The listing builds one solid part. Answer for the finished solid, in the listing's coordinates (mm). Give positions to 0.01 mm unless a question says otherwise; leave off trailing zeros. Write each loop counter-clockwise with the first axis right and the second up, starting at its lowest first coordinate (ties: lowest second). Pieces come first, ordered by that corner, then holes. Notation, with made-up numbers: (34.25, -37) - (46.25, -37) arc R19 ccw to (46.25, -24) - close; hole circle Ø1 at (43.25, -19). An arc over 180 degrees is marked (long way). Write each question's results on one line, items separated by ' | '. Start each with the question number.
Q1. For a pull along X with two mould halves and no side action, classify faces 1 (the face through (0, 0, 0)), 2 (the face through (-25.81, 0.49, 16.03)) as pulls with the +X half, pulls with the -X half, needs draft (parallel to the pull), parting line crosses it, or undercut.
Q2. Find the intervals of material crossed by probe 1 along Z at (x, y) = (-27, 0.6) (3 decimals); probe 2 along Z at (x, y) = (23, 1.3); probe 3 along X at (y, z) = (1.55, 9), in increasing order.
Q3. Section A-A (x = 27) is taken. Determine the outline of the cut face in (y, z) (3 decimals).
Q4. Section C-C (z = -1) is taken. Determine the outline of the cut face in (x, y) (3 decimals).
Q5. Section B-B (y = 1.5) is taken. Determine the outline of the cut face in (x, z).
Q6. Flat-ended cylindrical pins translate along their axes: pin 1 Ø1.8 at (x, z) = (27, 15.115) entering from -Y; pin 2 Ø0.5 at (y, z) = (1.5, 6) entering from -X; pin 3 Ø0.8 at (x, y) = (20.5, 1.5) entering from +Z; pin 4 Ø0.5 at (y, z) = (1.5, -2.5) entering from +X. Find the tip coordinate at first contact, or state that the pin passes through.
Q7. Section D-D (x = -5) is taken. Determine the outline of the cut face in (y, z) (3 decimals), plus the area to 4 significant figures.
```python
from build123d import *

# Parameters (mm, degrees)
SKETCH_2_W                = 60.73
SKETCH_2_H                = 36.85
EXTRUDE_1_DEPTH           = 1
HOLE_WIZARD_3_0_3_1_D     = 3
HOLE_WIZARD_3_0_3_1_DEPTH = 12.4
HOLE_WIZARD_3_0_3_1_TIP   = 0.901290929
SKETCH_6_W                = 7.681831357
SKETCH_6_H                = 4.985018222
SKETCH_6_W_2              = 7.845274578
SKETCH_6_H_2              = 4.821575001
EXTRUDE_2_DEPTH           = 1


with BuildPart() as part:
    # 草图2 → 凸台-拉伸1 (new body)
    with BuildSketch(Plane(origin=(0, 0, 0), x_dir=(1, 0, 0), z_dir=(0, 1, 0))):
        Rectangle(SKETCH_2_W, SKETCH_2_H)
    extrude(amount=EXTRUDE_1_DEPTH)

    # Ø3.0 (3) 直径孔1
    with Locations(Plane(origin=(0, 1, 0), x_dir=(1, 0, 0), z_dir=(0, 1, 0))):
        with Locations((-27, 15.115), (27, 15.115), (27, -15.115), (-27, -15.115)):
            Hole(HOLE_WIZARD_3_0_3_1_D / 2, depth=HOLE_WIZARD_3_0_3_1_DEPTH)
            with Locations((0, 0, -(HOLE_WIZARD_3_0_3_1_DEPTH + HOLE_WIZARD_3_0_3_1_TIP / 2))):  # 118° drill point
                Cone(0, HOLE_WIZARD_3_0_3_1_D / 2, HOLE_WIZARD_3_0_3_1_TIP, mode=Mode.SUBTRACT)

    # 草图6 → 凸台-拉伸2 (add)
    with BuildSketch(Plane(origin=(0, 1, 0), x_dir=(1, 0, 0), z_dir=(0, 1, 0))):
        with Locations((8.702195721, 1.796125826)):
            Rectangle(SKETCH_6_W, SKETCH_6_H)
        with Locations((19.652891485, 1.796125826)):
            Rectangle(SKETCH_6_W_2, SKETCH_6_H)
        with Locations((8.702195721, -6.866364854)):
            Rectangle(SKETCH_6_W, SKETCH_6_H_2)
        with Locations((19.652891485, -6.866364854)):
            Rectangle(SKETCH_6_W_2, SKETCH_6_H_2)
    extrude(amount=EXTRUDE_2_DEPTH)


solid = part.part
```
Answers below:
1) face 1: needs draft | face 2: undercut
2) probe 1: z = -18.425 to -16.615, -13.615 to 13.615, 16.615 to 18.425 | probe 2: z = -4.29 to 0.7, 4.46 to 9.28 | probe 3: x = 4.86 to 12.54, 15.73 to 23.58
3) outline: (0, -18.425) - (1, -18.425) - (1, -16.615) - (0, -16.615) - close; (0, -13.615) - (1, -13.615) - (1, 13.615) - (0, 13.615) - close; (0, 16.615) - (1, 16.615) - (1, 18.425) - (0, 18.425) - close
4) outline: (-30.365, 0) - (30.365, 0) - (30.365, 1) - (23.576, 1) - (23.576, 2) - (15.73, 2) - (15.73, 1) - (12.543, 1) - (12.543, 2) - (4.861, 2) - (4.861, 1) - (-30.365, 1) - close
5) outline: (4.86, -4.29) - (12.54, -4.29) - (12.54, 0.7) - (4.86, 0.7) - close; (4.86, 4.46) - (12.54, 4.46) - (12.54, 9.28) - (4.86, 9.28) - close; (15.73, -4.29) - (23.58, -4.29) - (23.58, 0.7) - (15.73, 0.7) - close; (15.73, 4.46) - (23.58, 4.46) - (23.58, 9.28) - (15.73, 9.28) - close
6) pin 1: passes through | pin 2: stops at x = 4.86 | pin 3: stops at z = 9.28 | pin 4: stops at x = 23.58
7) outline: (0, -18.425) - (1, -18.425) - (1, 18.425) - (0, 18.425) - close | area: 36.85 mm2
